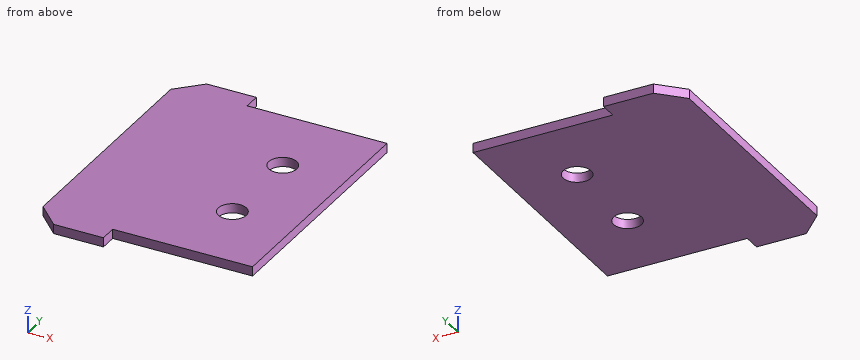
Autodesk Fusion 360 part; units mm, degrees
sketch "スケッチ1" plane through (0, 0, 0) normal (0, 0, 1) x (1, 0, 0)
  line L0 (-21.5, 91) -> (-68.5, 91)
  line L1 (-68.5, 91) -> (-68.5, -91)
  line L2 (-68.5, -91) -> (-21.5, -91)
  line L3 (68.5, -80) -> (68.5, 80)
  line L4 (60.2198, 80) -> (-68.5, -91) construction
  line L5 (-68.5, 91) -> (60.2198, -80) construction
  line L6 (-21.5, 91) -> (-21.5, 80)
  line L7 (-21.5, 80) -> (68.5, 80)
  line L8 (-21.5, -91) -> (-21.5, -80)
  line L9 (-21.5, -80) -> (68.5, -80)
  dimension "d2" = 182
extrude "押し出し1" add sketch "スケッチ1" along normal blind 6
chamfer "面取り1" distance 15 angle 45 2 edges at (-68.5, -91, 3) (-68.5, 91, 3)
sketch "スケッチ2" plane through (0, 0, 6) normal (0, 0, 1) x (-1, 0, 0)
  line L0 (53.5, -91) -> (68.5, -76)
  line L1 (68.5, -76) -> (68.5, 76)
  line L2 (68.5, 76) -> (53.5, 91)
  line L3 (53.5, 91) -> (21.5, 91)
  line L4 (21.5, 91) -> (21.5, 80)
  line L5 (21.5, 80) -> (-68.5, 80)
  line L6 (-68.5, 80) -> (-68.5, -80)
  line L7 (-68.5, -80) -> (21.5, -80)
  line L8 (21.5, -80) -> (21.5, -91)
  line L9 (21.5, -91) -> (53.5, -91)
  line L10 (-68.5, -80) -> (-28.5, -80) construction
  line L11 (-28.5, -80) -> (-28.5, -30) construction
  line L12 (-28.5, -30) -> (-68.5, -30) construction
  line L13 (-68.5, -30) -> (-68.5, -80) construction
  line L14 (-68.5, 0) -> (91.4537, 0)
  point P0 (-28.5, -30)
  point P1 (-28.5, 30)
  dimension "d10" = 40
  dimension "d11" = 50
hole "穴1" at (28.5, 30, 6) at (28.5, -30, 6) direction (0, 0, -1) diameter 18 end through all
Check sheet for the modelled part. Datum: model origin and axes. Units: mm. Coordinates: 2 decimals unless noted, no trailing zeros. Loops run counter-clockwise (first coordinate to the right, second up) from the corner with the lowest first, then second, coordinate; pieces in that order, holes last. Notation, with made-up numbers: M -21.5,66 L 36.5,66 A27 cw 36.5,98 Z; hole C -9.75,-6.75 d8. An arc over 180 degrees is marked long. Answer as a JSON object with one key per item and string values.
1. Sectioned sample at A-A on x = 28.5. Record the cut outline in (y, z), and give its area (3 significant figures).
Outcome:
{"outline": "M -80,0 L -39,0 L -39,6 L -80,6 Z; M -21,0 L 21,0 L 21,6 L -21,6 Z; M 39,0 L 80,0 L 80,6 L 39,6 Z", "area": "744 mm²"}
2. Depth check by flat-ended pin: P1, Ø23.5, axis at x = 28.5, y = 30, coming from the +Z side; P2, Ø3, axis at y = -84.5, z = 1.5, coming from the +X side; P3, Ø1.8, axis at x = 28, z = 2.5, coming from the -Y side. Enter the tip coordinate at first touch or a pass-through.
Outcome:
{"P1": "z = 6", "P2": "x = -21.5", "P3": "y = -80"}
3. Sectioned sample at D-D on y = 32.5. Record the cut outline in (x, z), and give its area (3 significant figures).
Outcome:
{"outline": "M -68.5,0 L 19.85,0 L 19.85,6 L -68.5,6 Z; M 37.15,0 L 68.5,0 L 68.5,6 L 37.15,6 Z", "area": "718 mm²"}
4. Scan lines: L1, parallel to Y at x = 28.5, z = 2.3; L2, parallel to Y at x = 33, z = 1.3; L3, parallel to X at y = 30, z = 1.3. Record each from-to range of solid material in increasing order. Write a range as from..to.
Outcome:
{"L1": "-80..-39, -21..21, 39..80", "L2": "-80..-37.79, -22.21..22.21, 37.79..80", "L3": "-68.5..19.5, 37.5..68.5"}
5. Sectioned sample at C-C on z = 1.75. Record the cut outline in (x, y), and give its area (3 significant figures).
Outcome:
{"outline": "M -68.5,-76 L -53.5,-91 L -21.5,-91 L -21.5,-80 L 68.5,-80 L 68.5,80 L -21.5,80 L -21.5,91 L -53.5,91 L -68.5,76 Z; hole C 28.5,-30 d18; hole C 28.5,30 d18", "area": "22,200 mm²"}
6. Sectioned sample at B-B on y = -30. Record the cut outline in (x, z), and give its area (3 significant figures).
Outcome:
{"outline": "M -68.5,0 L 19.5,0 L 19.5,6 L -68.5,6 Z; M 37.5,0 L 68.5,0 L 68.5,6 L 37.5,6 Z", "area": "714 mm²"}
